Can you work these out from the drawing? Everything is in mm from the part's minimum corner. Coordinates: 2 decimals unless noted, no trailing zeros. Loops run counter-clockwise (first coordinate to the right, second up) from the corner with the lowest first, then second, coordinate; pieces in that order, holes last. Notation, with made-up numbers: (66, 66.5) - (111, 66.5) arc R20 ccw to (111, 80.5) - close; hole circle Ø3 at (61, 83). An arc over 180 degrees is marked (long way). Put each result on its own line as item: value. Start each with the question number.
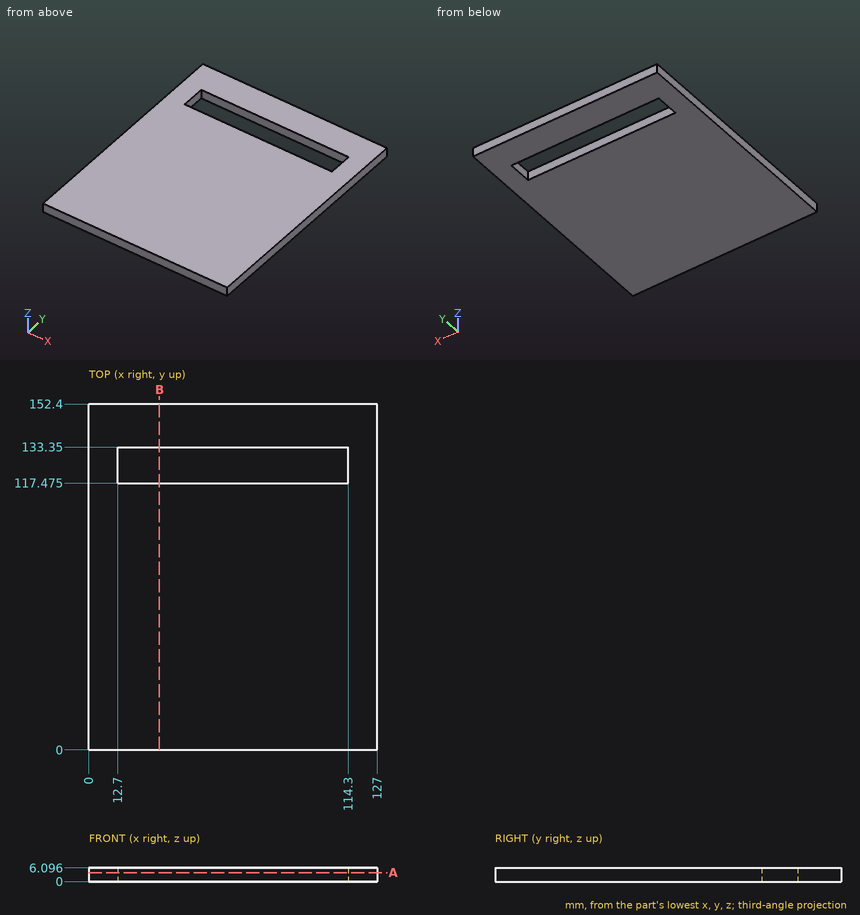
(1) For pin 1 Ø1.8 at (x, z) = (87.5, 4.5) entering from -Y, with a flat end and sliding along its axis, tell me the tip position at first contact or that it passes through.
(2) I want a section at A-A on z = 4. List the corners of the cut face in (x, y) for me (3 decimals).
(3) I need wall thicknesses on L1, parallel to Y at x = 29.5, z = 4.75 (3 decimals); L2, parallel to X at y = 118.5, z = 4.75. Which ranges of each line are inside material? Lowest first, please. Write a range as [from, to].
(4) I want a section at B-B on x = 31. List the corners of the cut face in (y, z) for me (3 decimals), and give its area (3 significant figures).
Answer sheet:
1. pin 1: stops at y = 0
2. outline: (0, 0) - (127, 0) - (127, 152.4) - (0, 152.4) - close; hole (12.7, 117.475) - (114.3, 117.475) - (114.3, 133.35) - (12.7, 133.35) - close
3. L1: y = [0, 117.475], [133.35, 152.4]
3. L2: x = [0, 12.7], [114.3, 127]
4. outline: (0, 0) - (117.475, 0) - (117.475, 6.096) - (0, 6.096) - close; (133.35, 0) - (152.4, 0) - (152.4, 6.096) - (133.35, 6.096) - close
4. area: 832 mm^2
